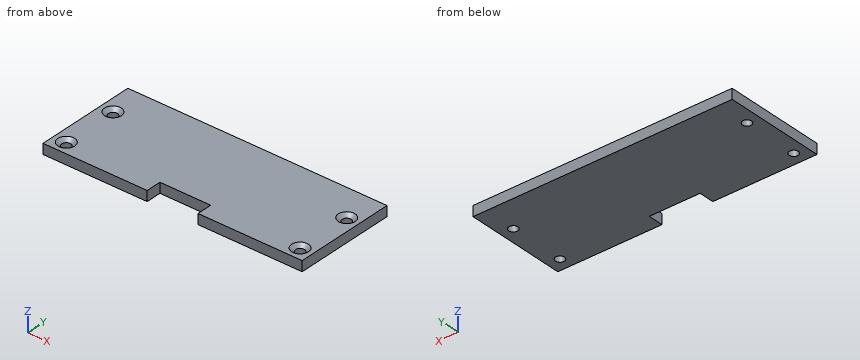
```python
from build123d import *

# Parameters (mm, degrees)
SKETCH1_W                                         = 129.54
SKETCH1_H                                         = 50.8
BOSS_EXTRUDE1_DEPTH                               = 5.08
CSK_FOR_8_FLAT_HEAD_MACHINE_SCREW_100_D           = 4.4958
CSK_FOR_8_FLAT_HEAD_MACHINE_SCREW_100_CSINK_D     = 8.4328
CSK_FOR_8_FLAT_HEAD_MACHINE_SCREW_100_CSINK_ANGLE = 100
SKETCH5_W                                         = 25.4
SKETCH5_H                                         = 7.62
CUT_EXTRUDE1_DEPTH                                = 6.08


with BuildPart() as part:
    # Sketch1 → Boss-Extrude1 (new body)
    with BuildSketch(Plane.XY):
        Rectangle(SKETCH1_W, SKETCH1_H)
    extrude(amount=BOSS_EXTRUDE1_DEPTH)

    # CSK for #8 Flat Head Machine Screw (100)1 (through all)
    with Locations(Plane.XY.offset(5.08)):
        with Locations((-58.42, 8.89), (-58.42, -19.05), (58.42, -19.05), (58.42, 8.89)):
            CounterSinkHole(CSK_FOR_8_FLAT_HEAD_MACHINE_SCREW_100_D / 2, CSK_FOR_8_FLAT_HEAD_MACHINE_SCREW_100_CSINK_D / 2, counter_sink_angle=CSK_FOR_8_FLAT_HEAD_MACHINE_SCREW_100_CSINK_ANGLE)

    # Sketch5 → Cut-Extrude1 (cut, through all)
    with BuildSketch(Plane.XY.offset(5.08)):
        with Locations((0, -21.59)):
            Rectangle(SKETCH5_W, SKETCH5_H)
    extrude(amount=-CUT_EXTRUDE1_DEPTH, mode=Mode.SUBTRACT)


solid = part.part
```
For this review, take the finished solid that the model builds, in its own axes (mm). Round coordinates to 2 decimals unless told otherwise and drop trailing zeros. Loops run counter-clockwise (first coordinate to the right, second up) from the corner with the lowest first, then second, coordinate; pieces in that order, holes last.
Q1. Add section B-B on z = 2.65. Write out the cut boundary in (x, y).
Result sheet:
outline: (-64.77, -25.4) - (-12.7, -25.4) - (-12.7, -17.78) - (12.7, -17.78) - (12.7, -25.4) - (64.77, -25.4) - (64.77, 25.4) - (-64.77, 25.4) - close; hole circle Ø4.5 at (-58.42, -19.05); hole circle Ø4.5 at (-58.42, 8.89); hole circle Ø4.5 at (58.42, -19.05); hole circle Ø4.5 at (58.42, 8.89)
Q2. Add section C-C on x = -58.42. Write out the cut boundary in (y, z), plus the area to 3 significant figures.
Result sheet:
outline: (-25.4, 0) - (-21.3, 0) - (-21.3, 3.43) - (-23.27, 5.08) - (-25.4, 5.08) - close; (-16.8, 0) - (6.64, 0) - (6.64, 3.43) - (4.67, 5.08) - (-14.83, 5.08) - (-16.8, 3.43) - close; (11.14, 0) - (25.4, 0) - (25.4, 5.08) - (13.11, 5.08) - (11.14, 3.43) - close
area: 206 mm2
Q3. Add section D-D on y = 8.89. Write out the cut boundary in (x, z).
Result sheet:
outline: (-64.77, 0) - (-60.67, 0) - (-60.67, 3.43) - (-62.64, 5.08) - (-64.77, 5.08) - close; (-56.17, 0) - (56.17, 0) - (56.17, 3.43) - (54.2, 5.08) - (-54.2, 5.08) - (-56.17, 3.43) - close; (60.67, 0) - (64.77, 0) - (64.77, 5.08) - (62.64, 5.08) - (60.67, 3.43) - close
Q4. To check wall thickness, follow line 1 along X through (y, z) = (-19.05, 1.75); line 2 along Y through (x, z) = (-58.42, 1.9); line 3 along X through (y, z) = (8.89, 1.05). State the ranges of each line that lie inside material, in increasing order.
Result sheet:
line 1: x = -64.77 to -60.67, -56.17 to -12.7, 12.7 to 56.17, 60.67 to 64.77
line 2: y = -25.4 to -21.3, -16.8 to 6.64, 11.14 to 25.4
line 3: x = -64.77 to -60.67, -56.17 to 56.17, 60.67 to 64.77
Q5. Add section A-A on y = -19.05. Write out the cut boundary in (x, z).
Result sheet:
outline: (-64.77, 0) - (-60.67, 0) - (-60.67, 3.43) - (-62.64, 5.08) - (-64.77, 5.08) - close; (-56.17, 0) - (-12.7, 0) - (-12.7, 5.08) - (-54.2, 5.08) - (-56.17, 3.43) - close; (12.7, 0) - (56.17, 0) - (56.17, 3.43) - (54.2, 5.08) - (12.7, 5.08) - close; (60.67, 0) - (64.77, 0) - (64.77, 5.08) - (62.64, 5.08) - (60.67, 3.43) - close
Q6. Insertion check: pin 1 Ø4 at (x, y) = (58.42, 8.89) entering from +Z; pin 2 Ø7 at (x, y) = (-58.42, -19.05) entering from +Z. Each pin has a flat end and moves straight along its axis. Give the tip position at first contact, or say it passes through.
Result sheet:
pin 1: passes through
pin 2: stops at z = 4.48
